```python
from build123d import *

# Parameters (mm, degrees)
EXTRUDE_1_DEPTH     = 15
SKETCH2_W           = 15
SKETCH2_H           = 15
EXTRUDE_2_DEPTH     = 65
SKETCH3_R           = 20
EXTRUDE_3_DEPTH     = 25
HOLE_WIZARD_1_D     = 20
HOLE_WIZARD_1_DEPTH = 25


with BuildPart() as part:
    # Sketch1 → 填料-伸長1 (new body)
    with BuildSketch(Plane(origin=(0, 0, 0), x_dir=(1, 0, 0), z_dir=(0, 1, 0))):
        with BuildLine():
            Line((32.5, 0), (32.5, 68))
            Line((32.5, 68), (-32.5, 68))
            Line((-32.5, 68), (-32.5, 0))
            ThreePointArc((-32.5, 0), (0, -32.5), (32.5, 0))
        make_face()
    extrude(amount=EXTRUDE_1_DEPTH)

    # Sketch2 → 填料-伸長2 (add, through all)
    with BuildSketch(Plane(origin=(32.5, 0, 0), x_dir=(0, 0, -1), z_dir=(1, 0, 0))):
        with Locations((60.5, -7.5)):
            Rectangle(SKETCH2_W, SKETCH2_H)
    extrude(amount=-EXTRUDE_2_DEPTH)

    # Sketch3 → 填料-伸長3 (add)
    with BuildSketch(Plane(origin=(0, 15, 0), x_dir=(-1, 0, 0), z_dir=(0, 1, 0))):
        with Locations(Location((0, 0, 0), (0, 0, 270))):
            Circle(SKETCH3_R)
    extrude(amount=EXTRUDE_3_DEPTH)

    # 鑽孔1
    with Locations(Plane(origin=(0, 40, 0), x_dir=(-1, 0, 0), z_dir=(0, 1, 0))):
        with Locations((0, 0)):
            Hole(HOLE_WIZARD_1_D / 2, depth=HOLE_WIZARD_1_DEPTH)


solid = part.part
```
The listing builds one solid part. Answer for the finished solid, in the listing's coordinates (mm). A direction names the side the tool comes from. Give positions to 0.01 mm unless a question says otherwise; leave off trailing zeros. Order: outer loops, then holes, each group sorted by start corner. A loop starts at its lowest first (then second) coordinate and runs counter-clockwise, first axis right, second up. Notation, with made-up numbers: (32, 39.5) - (41, 39.5) arc R7 ccw to (41, 50.5) - close; hole circle Ø2 at (-19, 46.5). An arc over 180 degrees is marked (long way). Use one line per item in the form item = value. Start each with the question number.
(1) A cutting plane is placed at B-B, the plane y = 21.5. Write down the section's boundary in (x, z).
(2) Flat-ended cylindrical pins translate along their axes: pin 1 Ø16 at (x, z) = (2, 4) entering from +Y; pin 2 Ø18 at (x, z) = (0, 0) entering from -Y; pin 3 Ø3 at (x, y) = (13.5, 20.5) entering from -Z; pin 4 Ø7.5 at (x, y) = (-0.5, -5.5) entering from +Z. Find the tip coordinate at first contact, or state that the pin passes through.
(3) A cutting plane is placed at C-C, the plane z = 6. Write down the section's boundary in (x, y).
(4) For faces 4 (the flat face through (0, 0, -11)), 5 (the cylindrical face through (19.524, 27.325, 4.336)), 6 (the flat face through (0, -15, -60)), determine the directions among +Z, -Z, +X, -X, +Y, -Y from which every point of the face is accessible in a straight line to the end or side of a thin tool.
(5) The mould has two halves that part along Z. Classify faces 1 (the flat face through (0, 15, 0)), 2 (the flat face through (32.5, 4, -41)), 3 (the flat face through (0, -8, -53)): released by +Z, released by -Z, zero draft, split by the parting line, or undercut.
(6) A cutting plane is placed at A-A, the plane x = 0. Write down the section's boundary in (y, z).
(7) Consider line 1 (Y direction, x = 21, z = -60.5); line 2 (Y direction, x = 14, z = -38); line 3 (Z direction, x = 0, y = 14). Determine where each line is inside the solid, lowest interval first. Write a range as from..to.
(8) A cutting plane is placed at D-D, the plane z = -22. Write down the section's boundary in (x, y).
Ans:
q1.outline = circle Ø40 at (0, 0); hole circle Ø20 at (0, 0)
q2.pin_1 = 40
q2.pin_2 = 0
q2.pin_3 = -16
q2.pin_4 = -53
q3.outline = (-31.94, 0) - (31.94, 0) - (31.94, 15) - (19.08, 15) - (19.08, 40) - (8, 40) - (8, 15) - (-8, 15) - (-8, 40) - (-19.08, 40) - (-19.08, 15) - (-31.94, 15) - close
q4.face_4 = +Z, +X, -X, -Y
q4.face_5 = +Y
q4.face_6 = +Z, -Z, +X, -X, -Y
q5.face_1 = undercut
q5.face_2 = zero draft
q5.face_3 = released by +Z
q6.outline = (-15, -68) - (15, -68) - (15, -20) - (40, -20) - (40, -10) - (15, -10) - (15, 10) - (40, 10) - (40, 20) - (15, 20) - (15, 32.5) - (0, 32.5) - (0, -53) - (-15, -53) - close
q7.line_1 = -15..15
q7.line_2 = 0..15
q7.line_3 = -68..32.5
q8.outline = (-32.5, 0) - (32.5, 0) - (32.5, 15) - (-32.5, 15) - close
